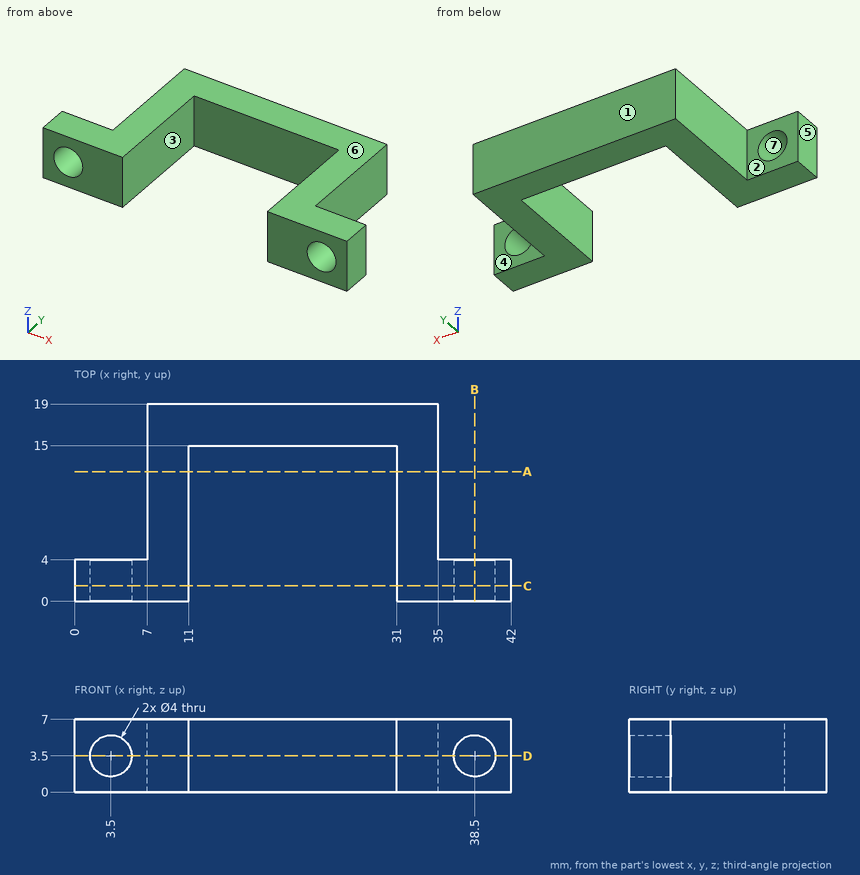
Could you check a few things on this drawing? It's one solid part, dimensions in mm from its lowest x, y, z. A direction names the side the tool comes from. Round coordinates to 2 decimals unless told otherwise and drop trailing zeros. Order: outer loops, then holes, each group sorted by start corner. A loop starts at its lowest first (then second) coordinate and runs counter-clockwise, first axis right, second up.
(1) Imagine slicing it at C-C (y = 1.5). Write out the boundary of the cut face in (x, z).
Response values:
outline: (0, 0) - (11, 0) - (11, 7) - (0, 7) - close; (31, 0) - (42, 0) - (42, 7) - (31, 7) - close; hole circle Ø4 at (3.5, 3.5); hole circle Ø4 at (38.5, 3.5)
(2) Imagine slicing it at D-D (z = 3.5). Write out the boundary of the cut face in (x, y).
Response values:
outline: (0, 0) - (1.5, 0) - (1.5, 4) - (0, 4) - close; (5.5, 0) - (11, 0) - (11, 15) - (31, 15) - (31, 0) - (36.5, 0) - (36.5, 4) - (35, 4) - (35, 19) - (7, 19) - (7, 4) - (5.5, 4) - close; (40.5, 0) - (42, 0) - (42, 4) - (40.5, 4) - close
(3) Which directions (+Z, -Z, +X, -X, +Y, -Y) give clear straight access to the entire face, cutting with the end or side of a thin tool? Please do the marked faces 1, 2, 3 and 4.
Response values:
face 1: +Z, -Z, +X, -X, +Y
face 2: +Z, -Z, -X, +Y
face 3: +Z, -Z, -Y
face 4: +Z, -Z, +X, +Y
(4) Please list where these lines run through material, in increasing order: line 1 along Z through (x, y) = (38.5, 2); line 2 along X through (y, z) = (7, 4.75); line 3 along Y through (x, z) = (30, 6).
Response values:
line 1: z = 0 to 1.5, 5.5 to 7
line 2: x = 7 to 11, 31 to 35
line 3: y = 15 to 19
(5) Imagine slicing it at A-A (y = 12.5). Write out the boundary of the cut face in (x, z), plus the area to 3 significant figures.
Response values:
outline: (7, 0) - (11, 0) - (11, 7) - (7, 7) - close; (31, 0) - (35, 0) - (35, 7) - (31, 7) - close
area: 56.0 mm2
(6) Imagine slicing it at B-B (x = 38.5). Write out the boundary of the cut face in (y, z), plus the area to 3 significant figures.
Response values:
outline: (0, 0) - (4, 0) - (4, 1.5) - (0, 1.5) - close; (0, 5.5) - (4, 5.5) - (4, 7) - (0, 7) - close
area: 12.0 mm2
(7) I'm going to push flat-ended pins straight in: pin 1 (3.5 mm diameter, centred on x = 3.5, z = 2, fed in from +Y); pin 2 (1 mm diameter, centred on y = 5.5, z = 2, fed in from -X); pin 3 (3.5 mm diameter, centred on y = 9, z = 3, fed in from +X); pin 4 (3 mm diameter, centred on x = 10.5, z = 3, fed in from -Y). Where does each tip first touch, or does it pass through?
Response values:
pin 1: stops at y = 4
pin 2: stops at x = 7
pin 3: stops at x = 35
pin 4: stops at y = 0
(8) If we mould it in two halves opening along Z, with no side actions, what happens to the marked faces 5, 6 and 7? For each: released by +Z, released by -Z, zero draft, split by the parting line, or undercut.
Response values:
face 5: zero draft
face 6: released by +Z
face 7: undercut
